Read the model definition and answer for the solid it produces. Units are mm, in the model's axes. A direction names the side the tool comes from. Coordinates: 2 decimals unless noted, no trailing zeros. Write each loop counter-clockwise with the first axis right and the second up, starting at its lowest first coordinate (ties: lowest second). Pieces come first, ordered by that corner, then holes. Notation, with made-up numbers: (48.25, -1.75) - (68.25, -1.75) arc R5 ccw to (68.25, 7.25) - close; hole circle Ø8 at (83.5, -40). An arc over 180 degrees is marked (long way). Use a Markdown table: item, result.
from build123d import *

# Parameters (mm, degrees)
F0_R     = 73.025
F1_DEPTH = 88.9
F0_R_2   = 123.825
F2_DEPTH = 19.05
F3_R     = 9.525
F4_DEPTH = 123.826


with BuildPart() as f1:
    # F0 (on Right) → F1 (new body)
    with BuildSketch(Plane.YZ):
        Circle(F0_R)
        with BuildLine():
            ThreePointArc((7.9375, 32.378774), (26.229805, 20.576352), (33.3375, 0))
            ThreePointArc((33.3375, 0), (-20.576352, -26.229805), (-7.9375, 32.378774))
            Line((-7.9375, 32.378774), (-7.9375, 38.1))
            Line((-7.9375, 38.1), (7.9375, 38.1))
            Line((7.9375, 38.1), (7.9375, 32.378774))
        make_face(mode=Mode.SUBTRACT)
    extrude(amount=F1_DEPTH)

    # F0 (on Right) → F2 (join)
    with BuildSketch(Plane.YZ):
        Circle(F0_R_2)
        Polygon((-101.6, -9.525), (-101.6, 9.525), (-82.55, 9.525), (-82.55, 0), (-82.55, -9.525), align=None, mode=Mode.SUBTRACT)
        Circle(F0_R, mode=Mode.SUBTRACT)
        Polygon((82.55, 0), (82.55, 9.525), (101.6, 9.525), (101.6, -9.525), (82.55, -9.525), align=None, mode=Mode.SUBTRACT)
    extrude(amount=F2_DEPTH)

    # F3 (on Top) → F4 (cut, through all)
    with BuildSketch(Plane.XY):
        with Locations((50.8, 0)):
            Circle(F3_R)
    extrude(amount=F4_DEPTH, mode=Mode.SUBTRACT)


solid = f1.part
(1) Straight lines are drawn through the part: L1, parallel to X at y = 0, z = 45 (3 decimals); L2, parallel to Y at x = 52.5, z = 2; L3, parallel to Z at x = 59, y = 0 (1 decimal). For each, find the intervals that lie inside material, in ascending order.
Report:
| item | result |
|---|---|
| L1 | x = 0 to 41.275, 60.325 to 88.9 |
| L2 | y = -73 to -33.28, 33.28 to 73 |
| L3 | z = -73 to -33.3 |
(2) A cutting plane is placed at D-D, the plane z = 45. Write down the section's boundary in (x, y) (3 decimals).
Report:
| item | result |
|---|---|
| outline | (0, -115.359) - (19.05, -115.359) - (19.05, -57.512) - (88.9, -57.512) - (88.9, 57.512) - (19.05, 57.512) - (19.05, 115.359) - (0, 115.359) - close; hole circle Ø19.05 at (50.8, 0) |
(3) A cutting plane is placed at A-A, the plane y = 0. Count the separate pieces of the cut face and the enclosed holes in it, and give its area (3 significant figures).
Report:
| item | result |
|---|---|
| separate pieces | 3 |
| enclosed holes | 0 |
| area | 7,900 mm² |
(4) Each of these flat-tipped pins is pushed along its axis until it touches: P1, Ø12, axis at x = 23.5, y = -55, coming from the +Z side; P2, Ø5, axis at x = 16, y = -4, coming from the -Z side; P3, Ø3, axis at x = 54, y = 25, coming from the -Z side. Where does it stop, or does it pass through?
Report:
| item | result |
|---|---|
| P1 | stops at z = 112.85 |
| P2 | stops at z = -123.82 |
| P3 | stops at z = -69.14 |
(5) For faces 1 (the flat face through (19.05, 53, -53)), 2 (the flat face through (22, 7.938, 35)), 3 (the flat face through (0, 26, -26)), determine the directions among +Z, -Z, +X, -X, +Y, -Y from which every point of the face is accessible in a straight line to the end or side of a thin tool.
Report:
| item | result |
|---|---|
| face 1 | +X |
| face 2 | +X, -X |
| face 3 | +Z, -Z, -X, +Y, -Y |
(6) A cutting plane is placed at C-C, the plane y = -87. Write down the section's boundary in (x, z) (3 decimals), and give its area (3 significant figures).
Report:
| item | result |
|---|---|
| outline | (0, -88.111) - (19.05, -88.111) - (19.05, -9.525) - (0, -9.525) - close; (0, 9.525) - (19.05, 9.525) - (19.05, 88.111) - (0, 88.111) - close |
| area | 2,990 mm² |
(7) The mould has two halves that part along Z. Classify faces 4 (the flat face through (9, -92, 9.525)), 5 (the cylindrical face through (59.885, 2.861, 52.199)), 6 (the cylindrical face through (53.486, 69.653, 21.935)): pulls with the +Z half, pulls with the -Z half, needs draft (parallel to the pull), parting line crosses it, or undercut.
Report:
| item | result |
|---|---|
| face 4 | undercut |
| face 5 | needs draft |
| face 6 | parting line crosses it |
(8) A cutting plane is placed at B-B, the plane z = 3. Write down the section's boundary in (x, y), and give its area (3 significant figures).
Report:
| item | result |
|---|---|
| outline | (0, -123.79) - (19.05, -123.79) - (19.05, -101.6) - (0, -101.6) - close; (0, -82.55) - (19.05, -82.55) - (19.05, -72.96) - (88.9, -72.96) - (88.9, -33.2) - (0, -33.2) - close; (0, 33.2) - (88.9, 33.2) - (88.9, 72.96) - (19.05, 72.96) - (19.05, 82.55) - (0, 82.55) - close; (0, 101.6) - (19.05, 101.6) - (19.05, 123.79) - (0, 123.79) - close |
| area | 8,280 mm² |
